Part model, mm, in its own coordinate system. A direction names the side the tool comes from. Round coordinates to 2 decimals unless told otherwise and drop trailing zeros. Loops run counter-clockwise (first coordinate to the right, second up) from the corner with the lowest first, then second, coordinate; pieces in that order, holes last.
(1) Probe probe 1 along Z at (x, y) = (0, 0.25); probe 2 along Z at (x, y) = (2, -2); probe 3 along Z at (x, y) = (-4.5, 0.5). List the from-to ranges inside material, lowest first.
(2) Mould opens along X. For faces 1 (the face through (-0.54, 0.07, -2.44)), 2 (the face through (0, -3, 4)) say: +X half, -X half, draft (parallel to the pull), parting line (faces both ways), or undercut.
(3) Tool access for faces 3 (the face through (-5.744, 0.042, -0.253)), 4 (the face through (0, 3, 4)): list every direction of +Z, -Z, +X, -X, +Y, -Y with a clear straight run to the whole face (end or side of a thin tool).
(4) Cut at A-A on z = 0. List the corners of the cut face in (x, y), then the cut area to 3 significant figures.
(5) Flat gauge pins, fed straight in: pin 1 (6.5 mm diameter, centred on x = 0, z = 0, fed in from +Y); pin 2 (1 mm diameter, centred on x = -4, z = -32, fed in from -Y); pin 3 (4 mm diameter, centred on x = 0, z = 22.5, fed in from +Y). Where does each tip first touch, or does it go through?
from build123d import *

# Parameters (mm, degrees)
SKETCH1_R             = 5.75
BOSS_EXTRUDE1_DEPTH   = 3
BOSS_EXTRUDE2_DEPTH   = 0.15
CIRPATTERN1_COUNT     = 2
SKETCH4_R             = 2.5
CUT_EXTRUDE1_DEPTH    = 7.0000001
CHAMFER1_SIZE         = 1
CHAMFER1_SIZE2        = 1.191753593
CHAMFER1_PART_2_SIZE  = 1
CHAMFER1_PART_2_SIZE2 = 1.191753593


with BuildPart() as part:
    # Sketch1 → Boss-Extrude1 (new body, symmetric)
    with BuildSketch(Plane(origin=(0, 0, 0), x_dir=(1, 0, 0), z_dir=(0, 1, 0))):
        Circle(SKETCH1_R)
    extrude(amount=BOSS_EXTRUDE1_DEPTH, both=True)

    # Sketch3 → Boss-Extrude2 (add, symmetric)
    with BuildSketch(Plane(origin=(0, 0, 0), x_dir=(0.974370065, -0.224951054, 0), z_dir=(-0.224951054, -0.974370065, 0))):
        with BuildLine():
            Line((-3.842130485, 3.401744966), (-6.87806753, 6.437682011))
            Line((-6.87806753, 6.437682011), (-6.87806753, 60.5))
            ThreePointArc((-6.87806753, 60.5), (-5.999387873, 62.621320344), (-3.87806753, 63.5))
            Line((-3.87806753, 63.5), (-3.193113424, 63.5))
            ThreePointArc((-3.193113424, 63.5), (-0.110101392, 62.436373561), (1.661241396, 59.698014726))
            add(Edge.make_bspline(
                [(1.661241396, 59.698014726), (9.030851791, 31.313089237), (4.404985301, 2.253493698)],
                knots=[0, 0, 0, 1, 1, 1], degree=2))
            add(Edge.make_bspline(
                [(-3.842130485, 3.401744966), (0.406766217, 7.300677946), (4.404985301, 2.253493698)],
                knots=[0, 0, 0, 1, 1, 1], degree=2))
        make_face()
    boss_extrude2 = extrude(amount=BOSS_EXTRUDE2_DEPTH, both=True)

    # CirPattern1: Boss-Extrude2 ×2 about axis
    cirpattern1_axis = Axis((0, 3, 0), (0, -1, 0))
    for i in range(1, CIRPATTERN1_COUNT):
        add(boss_extrude2.rotate(cirpattern1_axis, i * 360 / CIRPATTERN1_COUNT))

    # Sketch4 → Cut-Extrude1 (cut, through all)
    with BuildSketch(Plane.XZ.offset(3)):
        Circle(SKETCH4_R)
    extrude(amount=-CUT_EXTRUDE1_DEPTH, mode=Mode.SUBTRACT)

    # Chamfer1
    chamfer1_edges = [part.edges().sort_by_distance(p)[0] for p in [
        (-2.5, 3, 0),
    ]]
    chamfer1_side = [part.faces().sort_by_distance(p)[0] for p in [
        (-2.5, 0, 0),
    ]]
    chamfer(chamfer1_edges, length=CHAMFER1_SIZE, length2=CHAMFER1_SIZE2, reference=chamfer1_side[0])

    # Chamfer1 part 2
    chamfer1_part_2_edges = [part.edges().sort_by_distance(p)[0] for p in [
        (-2.5, -3, 0),
    ]]
    chamfer1_part_2_side = [part.faces().sort_by_distance(p)[0] for p in [
        (-5.58736544, -3, 0),
    ]]
    chamfer(chamfer1_part_2_edges, length=CHAMFER1_PART_2_SIZE, length2=CHAMFER1_PART_2_SIZE2, reference=chamfer1_part_2_side[0])


solid = part.part
Final values:
1. probe 1: z = -5.75 to -2.5, 2.5 to 5.75
1. probe 2: z = -5.39 to -1.76, 1.76 to 5.39
1. probe 3: z = -3.58 to 3.58
2. face 1: undercut
2. face 2: draft
3. face 3: none
3. face 4: +Z, -Z, +X, -X, +Y
4. outline: (-5.75, -3) - (-3.5, -3) - (-2.5, -1.81) - (-2.5, 2) - (-3.69, 3) - (-5.75, 3) - close; (2.5, -1.81) - (3.5, -3) - (5.75, -3) - (5.75, 3) - (3.69, 3) - (2.5, 2) - close
4. area: 36.6 mm2
5. pin 1: stops at y = 2.63
5. pin 2: stops at y = -1.19
5. pin 3: stops at y = 0.62
